```python
from build123d import *

# Parameters (mm, degrees)
SKETCH_2_R      = 79.5
SKETCH_3_R      = 50
SKETCH_4_W      = 60
SKETCH_4_H      = 40
EXTRUDE_1_DEPTH = 40.9
EXTRUDE_2_DEPTH = 10
SKETCH_6_R      = 6
EXTRUDE_3_DEPTH = 60


with BuildPart() as part:
    # 草图2 → 放样1 section 0
    with BuildSketch(Plane.XY):
        Circle(SKETCH_2_R)
    # 草图3 → 放样1 section 1
    with BuildSketch(Plane.XY.offset(20)):
        Circle(SKETCH_3_R)
    loft()

    # 草图4 → 凸台-拉伸1 (add)
    with BuildSketch(Plane.XY.offset(20)):
        Rectangle(SKETCH_4_W, SKETCH_4_H)
    extrude(amount=EXTRUDE_1_DEPTH)

    # 草图5 → 凸台-拉伸2 (add)
    with BuildSketch(Plane.ZY.offset(30)):
        with BuildLine():
            Line((20, 10), (40, 10))
            ThreePointArc((40, 10), (50, 0), (40, -10))
            Line((40, -10), (20, -10))
            Line((20, -10), (20, 10))
        make_face()
    extrude(amount=EXTRUDE_2_DEPTH)

    # 草图6 → 凸台-拉伸3 (add)
    with BuildSketch(Plane.ZY.offset(40)):
        with Locations((40, 0)):
            Circle(SKETCH_6_R)
    extrude(amount=EXTRUDE_3_DEPTH)


solid = part.part
```
Part model, mm, in its own coordinate system. A direction names the side the tool comes from. Round coordinates to 2 decimals unless told otherwise and drop trailing zeros. Write each loop counter-clockwise with the first axis right and the second up, starting at its lowest first coordinate (ties: lowest second). Pieces come first, ordered by that corner, then holes.
Item 1: Drop flat-ended pins along their axis: pin 1 Ø2 at (x, y) = (12, 36) entering from +Z; pin 2 Ø11 at (x, z) = (-34, 32.5) entering from +Y; pin 3 Ø2 at (x, y) = (-25, -54.5) entering from +Z. Give the stop position or say it passes through.
Results:
pin 1: stops at z = 20
pin 2: stops at y = 20
pin 3: stops at z = 13.93
Item 2: Cut at C-C, the plane z = 12. Give the cut face in (x, y), plus the area to 3 significant figures.
Results:
outline: circle Ø123.6 at (0, 0)
area: 12,000 mm2
Item 3: Cut at B-B, the plane x = -86.5. Give the cut face in (y, z).
Results:
outline: circle Ø12 at (0, 40)
Item 4: Which spindle directions (+Z, -Z, +X, -X, +Y, -Y) get a long thin tool onto all of the face, cutting with end or side? Do faces 5 (the flat face through (-40, 0, 32)), 6 (the flat face through (-30, -5, 49)), 7 (the flat face through (30, 0, 40)), 8 (the flat face through (0, -20, 40)), 9 (the flat face through (0, 20, 40)). Say none if no direction does.
Results:
face 5: -X
face 6: +Z, -X
face 7: +Z, +X, +Y, -Y
face 8: +Z, +X, -X, -Y
face 9: +Z, +X, -X, +Y
Item 5: Probe L1, parallel to Z at x = 26, y = -24; L2, parallel to Y at x = 14.5, z = 35; L3, parallel to Y at x = -32, z = 32. List the from-to ranges inside material, lowest first.
Results:
L1: z = 0 to 20
L2: y = -20 to 20
L3: y = -10 to 10
Item 6: Two-plate mould, pull along Z, no slides. Class faces 1 (the cylindrical face through (-70, 0, 34)), 2 (the flat face through (-1, 1, 0)), 3 (the flat face through (-100, 0, 40)), 4 (the cylindrical face through (-35, 0, 50)): +Z half, -Z half, draft (parallel to the pull), parting line (faces both ways), or undercut.
Results:
face 1: undercut
face 2: -Z half
face 3: draft
face 4: +Z half
Item 7: Cut at A-A, the plane z = 22. Give the cut face in (x, y).
Results:
outline: (-40, -10) - (-30, -10) - (-30, -20) - (30, -20) - (30, 20) - (-30, 20) - (-30, 10) - (-40, 10) - close
